The model under review builds one solid part; all positions refer to its coordinate system, in mm. A direction names the side the tool comes from. Give positions to 0.01 mm unless a question says otherwise; leave off trailing zeros. Loops run counter-clockwise (first coordinate to the right, second up) from the corner with the lowest first, then second, coordinate; pieces in that order, holes last. Notation, with made-up numbers: M 82,25.5 L 124,25.5 A19 ccw 124,52.5 Z; hole C -12,66 d2. An arc over 180 degrees is marked long. Write item = value, one per line. Start each with the question number.
1. For faces 1 (the face through (28, 15, -11)), 2 (the face through (0, 28.25, 5)), 3 (the face through (-37.71, -1.73, -28.81)), 4 (the face through (37.79, -1.73, -28.81)), list the 3-axis set-ups (+Z, -Z, +X, -X, +Y, -Y) from which the entire face can be reached by the end or side of a thin tool; tool diameter is ignored.
2. We need section B-B on x = 28.25. Give the boundary of the cut face in (y, z), then the cut area to 3 significant figures.
3. Draft analysis for pull direction X (two halves, no side actions). For faces 5 (the face through (-24.09, 26.53, 5.58)), 6 (the face through (20, 0, -10)), 7 (the face through (-27, 0, -36)), 8 (the face through (42.5, 0, -21)), state which applies: pulls with the +X half, pulls with the -X half, needs draft (parallel to the pull), parting line crosses it, or undercut.
4. We need section D-D on y = 0. Give the boundary of the cut face in (x, z).
5. Wall thickness on line 1 along Y through (x, z) = (-28, 7); line 2 along Z through (x, y) = (-4.5, 8.5): over which ranges is each line inside the solid? List them lowest first. Write a range as from..to.
6. For pin 1 (7.5 mm diameter, centred on x = -27.5, z = -15.5, fed in from +Y); pin 2 (3 mm diameter, centred on x = 28, y = 8, fed in from -Z); pin 3 (1.5 mm diameter, centred on x = 29, z = -21.5, fed in from -Y); pin 4 (7 mm diameter, centred on x = 28.25, y = -28.25, fed in from +Z), all flat-tipped, find the tip position at first contact; note any pin that passes through.
7. We need section C-C on z = 1. Give the boundary of the cut face in (x, y).
8. We need section A-A on z = -30. Give the boundary of the cut face in (x, y).
from build123d import *

# Parameters (mm, degrees)
F1_DEPTH  = 11
F2_R      = 4.5
F3_DEPTH  = 11
F5_R      = 8
F6_DEPTH  = 70
F7_W      = 40
F7_H      = 30
F8_DEPTH  = 36.001
F9_R      = 8
F10_DEPTH = 42.5
F11_SIZE  = 2


with BuildPart() as f1:
    # F0 (on Top) → F1 (new body)
    with BuildSketch(Plane.XY):
        with BuildLine():
            Line((21.5, 28.25), (-21.5, 28.25))
            ThreePointArc((-21.5, 28.25), (-28.25, 35), (-35, 28.25))
            Line((-35, 28.25), (-35, -28.25))
            ThreePointArc((-35, -28.25), (-28.25, -35), (-21.5, -28.25))
            Line((-21.5, -28.25), (21.5, -28.25))
            ThreePointArc((21.5, -28.25), (28.25, -35), (35, -28.25))
            Line((35, -28.25), (35, 28.25))
            ThreePointArc((35, 28.25), (28.25, 35), (21.5, 28.25))
        make_face()
    extrude(amount=F1_DEPTH)

    # F2 (on face) → F3 (cut, through all)
    with BuildSketch(Plane.XY.offset(11)):
        with Locations((-28.25, 28.25)):
            Circle(F2_R)
        with Locations((28.25, 28.25)):
            Circle(F2_R)
        with Locations((28.25, -28.25)):
            Circle(F2_R)
        with Locations((-28.25, -28.25)):
            Circle(F2_R)
    extrude(amount=-F3_DEPTH, mode=Mode.SUBTRACT)

    # F5 (on offset) → F6 (join, through all)
    with BuildSketch(Plane.YZ.offset(35)):
        with BuildLine():
            Line((15, -21), (15, 0))
            Line((15, 0), (-15, 0))
            Line((-15, 0), (-15, -21))
            ThreePointArc((-15, -21), (0, -36), (15, -21))
        make_face()
        with Locations((0, -21)):
            Circle(F5_R, mode=Mode.SUBTRACT)
    extrude(amount=-F6_DEPTH)

    # F7 (on face) → F8 (cut, through all)
    with BuildSketch(Plane(origin=(0, 0, 0), x_dir=(1, 0, 0), z_dir=(0, 0, -1))):
        Rectangle(F7_W, F7_H)
    extrude(amount=F8_DEPTH, mode=Mode.SUBTRACT)

    # F9 (on Right) → F10 (join, symmetric)
    with BuildSketch(Plane.YZ):
        with Locations((0, -21)):
            Circle(F9_R)
    extrude(amount=F10_DEPTH, both=True)

    # F11
    f11_edges = [f1.edges().sort_by_distance(p)[0] for p in [
        (42.5, -8, -21),
        (-42.5, -8, -21),
    ]]
    chamfer(f11_edges, length=F11_SIZE)


solid = f1.part
Final values:
q1.face_1 = -Z, +X, -X, +Y
q1.face_2 = +Z, -Z, +Y
q1.face_3 = -X
q1.face_4 = +X
q2.outline = M -35,0 L -32.75,0 L -32.75,11 L -35,11 Z; M -23.75,0 L -15,0 L -15,-21 A15 ccw 15,-21 L 15,0 L 23.75,0 L 23.75,11 L -23.75,11 Z; M 32.75,0 L 35,0 L 35,11 L 32.75,11 Z
q2.area = 1,560 mm²
q3.face_5 = undercut
q3.face_6 = undercut
q3.face_7 = needs draft
q3.face_8 = pulls with the +X half
q4.outline = M -42.5,-27 L -40.5,-29 L -35,-29 L -35,-36 L -20,-36 L -20,-29 L 20,-29 L 20,-36 L 35,-36 L 35,-29 L 40.5,-29 L 42.5,-27 L 42.5,-15 L 40.5,-13 L 35,-13 L 35,11 L -35,11 L -35,-13 L -40.5,-13 L -42.5,-15 Z; hole M -20,-13 L 20,-13 L 20,0 L -20,0 Z
q5.line_1 = -35..-32.74, -23.76..23.76, 32.74..35
q5.line_2 = 0..11
q6.pin_1 = 15
q6.pin_2 = -34.52
q6.pin_3 = -15
q6.pin_4 = through
q7.outline = M -35,-28.25 A6.75 ccw -21.5,-28.25 L 21.5,-28.25 A6.75 ccw 35,-28.25 L 35,28.25 A6.75 ccw 21.5,28.25 L -21.5,28.25 A6.75 ccw -35,28.25 Z; hole C -28.25,-28.25 d9; hole C -28.25,28.25 d9; hole C 28.25,-28.25 d9; hole C 28.25,28.25 d9
q8.outline = M -35,-12 L -20,-12 L -20,12 L -35,12 Z; M 20,-12 L 35,-12 L 35,12 L 20,12 Z
